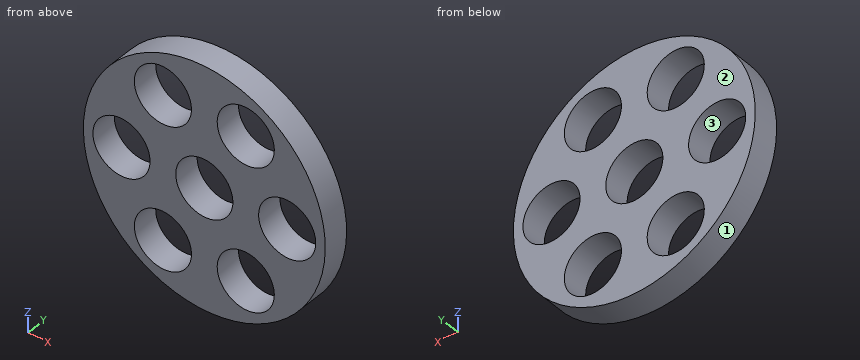
```python
from build123d import *

# Parameters (mm, degrees)
ESBO_O1_R                = 31.75
RESSALTO_EXTRUS_O1_DEPTH = 7
ESBO_O2_R                = 7.5
CORTE_EXTRUS_O1_DEPTH    = 10


with BuildPart() as part:
    # Esboço1 → Ressalto-extrusão1 (new body)
    with BuildSketch(Plane(origin=(0, 0, 0), x_dir=(1, 0, 0), z_dir=(0, 1, 0))):
        with Locations(Location((0, 0, 0), (0, 0, 270))):
            Circle(ESBO_O1_R)
    extrude(amount=-RESSALTO_EXTRUS_O1_DEPTH)

    # Esboço2 → Corte-extrusão1 (cut)
    with BuildSketch(Plane(origin=(0, 0, 0), x_dir=(1, 0, 0), z_dir=(0, 1, 0))):
        with Locations(Location((21.75, 0, 0), (0, 0, 270))):
            Circle(ESBO_O2_R)
        with Locations(Location((10.8755, -18.835186507, 0), (0, 0, 270))):
            Circle(ESBO_O2_R)
        with Locations(Location((-10.8735, -18.835186507, 0), (0, 0, 270))):
            Circle(ESBO_O2_R)
        with Locations(Location((-21.748, 0, 0), (0, 0, 270))):
            Circle(ESBO_O2_R)
        with Locations(Location((0.0015, -0.000866025, 0), (0, 0, 270))):
            Circle(ESBO_O2_R)
        with Locations(Location((-10.8735, 18.835186507, 0), (0, 0, 270))):
            Circle(ESBO_O2_R)
        with Locations(Location((10.8755, 18.835186507, 0), (0, 0, 270))):
            Circle(ESBO_O2_R)
    extrude(amount=-CORTE_EXTRUS_O1_DEPTH, mode=Mode.SUBTRACT)


solid = part.part
```
The listing builds one solid part. Answer for the finished solid, in the listing's coordinates (mm). Face numbers are marked on the shaded views. Give positions to 0.01 mm unless a question says otherwise; leave off trailing zeros. Write each loop counter-clockwise with the first axis right and the second up, starting at its lowest first coordinate (ties: lowest second). Pieces come first, ordered by that corner, then holes. Notation, with made-up numbers: (47, 18) -> (55, 18) arc R21 cw to (55, 42) -> close; hole circle Ø11 at (-5.5, 87). An arc over 180 degrees is marked (long way). Use one line per item in the form item = value.
1) Section B-B on z = 17 is taken. Write down the section's boundary in (x, y).
Result:
outline = (-26.82, -7) -> (-18.15, -7) -> (-18.15, 0) -> (-26.82, 0) -> close; (-3.6, -7) -> (3.6, -7) -> (3.6, 0) -> (-3.6, 0) -> close; (18.15, -7) -> (26.82, -7) -> (26.82, 0) -> (18.15, 0) -> close
2) Section C-C on x = 21.75 is taken. Write down the section's boundary in (y, z), plus the area to 3 significant figures.
Result:
outline = (-7, -23.13) -> (0, -23.13) -> (0, -7.5) -> (-7, -7.5) -> close; (-7, 7.5) -> (0, 7.5) -> (0, 23.13) -> (-7, 23.13) -> close
area = 219 mm²
3) Section A-A on z = 1.5 is taken. Write down the section's boundary in (x, y), plus the area to 3 significant figures.
Result:
outline = (-31.71, -7) -> (-29.1, -7) -> (-29.1, 0) -> (-31.71, 0) -> close; (-14.4, -7) -> (-7.35, -7) -> (-7.35, 0) -> (-14.4, 0) -> close; (7.35, -7) -> (14.4, -7) -> (14.4, 0) -> (7.35, 0) -> close; (29.1, -7) -> (31.71, -7) -> (31.71, 0) -> (29.1, 0) -> close
area = 135 mm²
4) Each of these flat-tipped pins is pushed along its axis until it touches: P1, Ø3, axis at x = -8, y = -6, coming from the +Z side; P2, Ø4, axis at x = 15.5, y = -5, coming from the +Z side; P3, Ø3, axis at y = -1, z = -15, coming from the -X side. Where does it stop, or does it pass through?
Result:
P1 = 31.08
P2 = 28.74
P3 = -28.74
5) For a pull along X with two mould halves and no side action, classify the marked faces 1, 2 and 3 as +X half, -X half, draft (parallel to the pull), parting line (faces both ways), or undercut.
Result:
face_1 = parting line
face_2 = draft
face_3 = undercut
6) Section D-D on y = -3 is taken. Write down the section's boundary in (x, z).
Result:
outline = circle Ø63.5 at (0, 0); hole circle Ø15 at (-21.75, 0); hole circle Ø15 at (-10.87, -18.84); hole circle Ø15 at (-10.87, 18.84); hole circle Ø15 at (0, 0); hole circle Ø15 at (10.88, -18.84); hole circle Ø15 at (10.88, 18.84); hole circle Ø15 at (21.75, 0)
7) Straight lines are drawn through the part: probe 1 along X at (y, z) = (-2.5, 0); probe 2 along X at (y, z) = (-4.5, 23); probe 3 along X at (y, z) = (-1, -5). For each, find the intervals that lie inside material, in ascending order.
Result:
probe_1 = -31.75 to -29.25, -14.25 to -7.5, 7.5 to 14.25, 29.25 to 31.75
probe_2 = -21.89 to -17.11, -4.64 to 4.64, 17.11 to 21.89
probe_3 = -31.35 to -27.34, -16.16 to -5.59, 5.59 to 16.16, 27.34 to 31.35
